For this review, take the finished solid that the model builds, in its own axes (mm). Face numbers are marked on the shaded views. A direction names the side the tool comes from. Round coordinates to 2 decimals unless told otherwise and drop trailing zeros. Write each loop counter-clockwise with the first axis right and the second up, starting at its lowest first coordinate (ties: lowest second). Pieces come first, ordered by that corner, then holes. Notation, with made-up numbers: (-31, 5) - (21, 5) arc R34 ccw to (21, 43) - close; hole circle Ø11 at (20, 29). An arc over 180 degrees is marked (long way). One line per item, written item: value. Start each with the question number.
Q1. Add section C-C on y = -44. Write out the cut boundary in (x, z).
Q2. Tool access review of the marked faces 1, 2 and 3: name each direction out of +Z, -Z, +X, -X, +Y, -Y from which nothing blocks a thin tool from reaching the whole face with its end or side.
Q3. Add section A-A on y = 32.5. Write out the cut boundary in (x, z), and give its area (3 significant figures).
Q4. Mouldability with a two-part tool opening along Y and no side actions: class the marked faces 4, 5 and 6 as +Y half, -Y half, draft (parallel to the pull), parting line (faces both ways), or undercut.
Q5. Add section B-B on z = 13. Write out the cut boundary in (x, y), and give its area (3 significant figures).
Q6. Clearance check with flat-ended pins moving along their axes: pin 1 Ø7 at (x, y) = (-5, -65) entering from +Z; pin 2 Ø4 at (x, z) = (-1.5, 16.5) entering from +Y; pin 3 Ø6.5 at (x, z) = (-4.5, 19.5) entering from -Y. State where each tip first meets the part, or that it passes through.
Q7. For probe 1 along Y at (x, z) = (-7, 0.55); probe 2 along Y at (x, z) = (-12, 45.5); probe 3 along Y at (x, z) = (-2.25, 20.5), list the stretches that pass through material, from the lowest coordinate up.
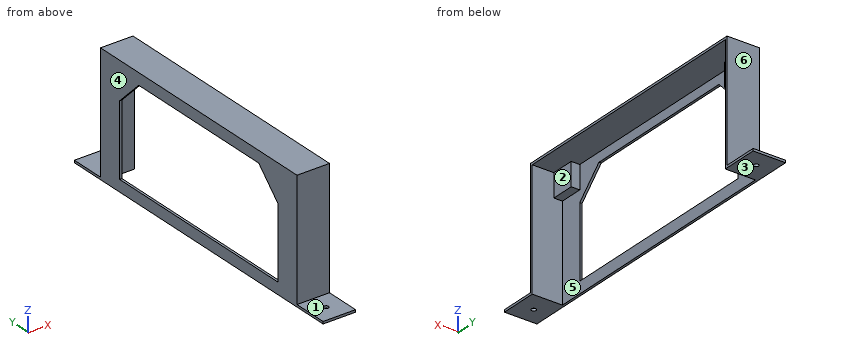
```python
from build123d import *

# Parameters (mm, degrees)
F0_W     = 14
F0_H     = 113
F1_DEPTH = 52
F2_W     = 13
F2_H     = 111
F3_DEPTH = 51
F4_W     = 14
F4_H     = 15
F4_R     = 1
F5_DEPTH = 1
F7_DEPTH = 1
F8_W     = 10
F8_H     = 10
F9_DEPTH = 3.7


with BuildPart() as f1:
    # F0 (on Top) → F1 (new body)
    with BuildSketch(Plane.XY):
        with Locations((-7, 0)):
            Rectangle(F0_W, F0_H)
    extrude(amount=F1_DEPTH)

    # F2 (on face) → F3 (cut)
    with BuildSketch(Plane(origin=(0, 0, 0), x_dir=(1, 0, 0), z_dir=(0, 0, -1))):
        with Locations((-6.5, 0)):
            Rectangle(F2_W, F2_H)
    extrude(amount=-F3_DEPTH, mode=Mode.SUBTRACT)

    # F4 (on Top) → F5 (join)
    with BuildSketch(Plane.XY):
        with Locations((-7, 64)):
            Rectangle(F4_W, F4_H)
        with Locations((-7, 64)):
            Circle(F4_R, mode=Mode.SUBTRACT)
        with Locations((-7, -64)):
            Rectangle(F4_W, F4_H)
        with Locations((-7, -64)):
            Circle(F4_R, mode=Mode.SUBTRACT)
    extrude(amount=F5_DEPTH)

    # F6 (on face) → F7 (cut)
    with BuildSketch(Plane.YZ.offset(-13)):
        Polygon((-45.5, 36), (-45.5, 5), (45.5, 5), (45.5, 36), (34.5, 47), (-34.5, 47), align=None)
    extrude(amount=-F7_DEPTH, mode=Mode.SUBTRACT)

    # F8 (on face) → F9 (join)
    with BuildSketch(Plane.YZ.offset(-13)):
        with Locations((-50.5, 46)):
            Rectangle(F8_W, F8_H)
        with Locations((47.5, 46)):
            Rectangle(F8_W, F8_H)
    extrude(amount=F9_DEPTH)


solid = f1.part
```
Result set:
1. outline: (-14, 0) - (-13, 0) - (-13, 5) - (-14, 5) - close; (-14, 37.5) - (-13, 37.5) - (-13, 51) - (0, 51) - (0, 52) - (-14, 52) - close
2. face 1: +Z, +X, -X, -Y
2. face 2: -Z, +X
2. face 3: -Z, +X, -X, +Y, -Y
3. outline: (-14, 0) - (-13, 0) - (-13, 5) - (-14, 5) - close; (-14, 47) - (-13, 47) - (-13, 51) - (0, 51) - (0, 52) - (-14, 52) - close
3. area: 23.0 mm^2
4. face 4: draft
4. face 5: undercut
4. face 6: +Y half
5. outline: (-14, -56.5) - (0, -56.5) - (0, -55.5) - (-13, -55.5) - (-13, -45.5) - (-14, -45.5) - close; (-14, 45.5) - (-13, 45.5) - (-13, 55.5) - (0, 55.5) - (0, 56.5) - (-14, 56.5) - close
5. area: 48.0 mm^2
6. pin 1: stops at z = 1
6. pin 2: stops at y = 56.5
6. pin 3: stops at y = -56.5
7. probe 1: y = -71.5 to -65, -63 to -55.5, 55.5 to 63, 65 to 71.5
7. probe 2: y = -56.5 to -45.5, 42.5 to 52.5, 55.5 to 56.5
7. probe 3: y = -56.5 to -55.5, 55.5 to 56.5
